Could you check a few things on this model? Use its own coordinates, in mm. A direction names the side the tool comes from. Give positions to 0.01 mm unless a question says otherwise; leave off trailing zeros. Order: outer loops, then holes, each group sorted by start corner. A loop starts at its lowest first (then second) coordinate and runs counter-clockwise, first axis right, second up. Notation, with made-up numbers: (45.5, 68.25) -> (101.5, 68.25) arc R21 ccw to (101.5, 90.25) -> close; hole circle Ø3 at (22.5, 80). An arc over 180 degrees is marked (long way). Answer as CSV lines item,"result". Start each with the question number.
(1) I need wall thicknesses on L1, parallel to Z at x = -55, y = 48.5; L2, parallel to Z at x = -57, y = 41; L3, parallel to Y at x = -1.5, z = -22.5. Which ranges of each line are inside material? Lowest first, please.
(2) I want a section at A-A (z = -12). Please give me the cut outline in (x, y), plus the area to 3 significant figures.
(3) We'd pull the mould along X, two halves only. Please class faces 4 (the face through (-62, 34, -25.6)), 5 (the face through (-69.42, -28.78, -13.04)), 6 (the face through (13.906, -62.625, -30.96)): released by +X, released by -X, zero draft, split by the parting line, or undercut.
(4) I want a section at B-B (z = -52.5). Please give me the cut outline in (x, y).
(5) On a 3-axis mill with a long thin cutter (end or side, diameter ignored), from which of +Z, -Z, +X, -X, +Y, -Y can I reach the whole of each face in a straight line? I mean faces 1 (the face through (-62, 34, -41.2)), 2 (the face through (-60.208, -46.166, -1.016)), 3 (the face through (-69.42, -28.78, -59.84)). Say none if no direction works.
(6) Will these pins go through, and if not, where does the flat tip stop? pin 1 Ø1 at (y, z) = (11.5, -13) entering from -X; pin 2 Ø2 at (x, y) = (46.73, -64.32) entering from -Z; pin 3 Ø6 at (y, z) = (35.5, -50.5) entering from +X; pin 4 Ø6 at (y, z) = (-11, -50.5) entering from -X.
```python
from build123d import *

# Parameters (mm, degrees)
M3X0_5_TAPPED_HOLE1_D = 2.5
SKETCH5_R             = 75.87
SKETCH5_R_2           = 72.77
CUT_EXTRUDE1_DEPTH    = 2.06


with BuildPart() as part:
    # Sketch1 → Revolve1 (revolve)
    with BuildSketch(Plane(origin=(0, 0, 0), x_dir=(1, 0, 0), z_dir=(0, 1, 0))):
        Polygon((-82.55, 0), (-82.55, 10), (-75.15, 10), (-75.15, 16), (-70.15, 16), (-70.15, 25.6), (-75.15, 25.6), (-75.15, 31.6), (-70.15, 31.6), (-70.15, 41.2), (-75.15, 41.2), (-75.15, 47.2), (-70.15, 47.2), (-70.15, 56.8), (-75.15, 56.8), (-75.15, 62.8), (-64.15, 62.8), (-64.15, 0), align=None)
    revolve(axis=Axis((0, 0, 0), (0, 0, -1)))

    # M3x0.5 Tapped Hole1 (through all)
    with Locations(Plane.XY):
        with Locations((0, 79.5), (46.728927557, 64.316851053), (75.608993045, 24.566851053), (75.608993045, -24.566851053), (46.728927557, -64.316851053), (0, -79.5), (-46.728927557, -64.316851053), (-75.608993045, -24.566851053), (-75.608993045, 24.566851053), (-46.728927557, 64.316851053)):
            Hole(M3X0_5_TAPPED_HOLE1_D / 2)

    # Sketch5 → Cut-Extrude1 (cut)
    with BuildSketch(Plane.XY):
        Circle(SKETCH5_R)
        Circle(SKETCH5_R_2, mode=Mode.SUBTRACT)
    extrude(amount=-CUT_EXTRUDE1_DEPTH, mode=Mode.SUBTRACT)


solid = part.part
```
Final values:
1,L1,"-62.8 to -56.8, -47.2 to -41.2, -31.6 to -25.6, -16 to -2.06"
1,L2,"-62.8 to -56.8, -47.2 to -41.2, -31.6 to -25.6, -16 to 0"
1,L3,"-70.13 to -64.13, 64.13 to 70.13"
2,outline,"circle Ø150.3 at (0, 0); hole circle Ø128.3 at (0, 0)"
2,area,"4,810 mm²"
3,face 4,"zero draft"
3,face 5,"split by the parting line"
3,face 6,"undercut"
4,outline,"circle Ø140.3 at (0, 0); hole circle Ø128.3 at (0, 0)"
5,face 1,"none"
5,face 2,"+Z"
5,face 3,"-Z"
6,pin 1,"x = -74.34"
6,pin 2,"through"
6,pin 3,"x = 62.17"
6,pin 4,"x = -69.69"
